Model file for the job. Use its own axes, mm. A direction names the side the tool comes from. Coordinates: 2 decimals unless noted, no trailing zeros. Write each loop counter-clockwise with the first axis right and the second up, starting at its lowest first coordinate (ties: lowest second). Pieces come first, ordered by that corner, then holes.
Q1. Pull direction Y, two halves, no side cores. Call faces 1 (the flat face through (1, 27, 228.6)), 2 (the cylindrical face through (24.6, 15.5, 11.2)), 3 (the flat face through (13, 50.8, 113)), 4 (the cylindrical face through (24.595, 35.423, 214.193)): released by +Y, released by -Y, zero draft, split by the parting line, or undercut.
Q2. Pin check, flat tip, straight feed: P1, Ø4, axis at y = 38.1, z = 215.9, coming from the -X side. Stop position of the tip, or through.
Q3. Drill centre lines: probe 1 along Z at (x, y) = (0.6, 38.1) (3 decimals); probe 2 along Y at (x, z) = (0.6, 12.7) (3 decimals); probe 3 along X at (y, z) = (37, 45). Where is each one in solid material? Low to high.
Q4. Band-saw the part on D-D, the plane x = 13.5. Write the cut outline in (y, z).
Q5. Band-saw the part on A-A, the plane y = 38.1. Write the cut outline in (x, z) (1 decimal), plus the area to 3 significant figures.
Q6. Band-saw the part on B-B, the plane z = 114.5. Write the cut outline in (x, y), plus the area to 3 significant figures.
Q7. Band-saw the part on C-C, the plane y = 25. Write the cut outline in (x, z), plus the area to 3 significant figures.
Q8. Which spindle directions (+Z, -Z, +X, -X, +Y, -Y) get a long thin tool onto all of the face, cutting with end or side? Do faces 5 (the flat face through (13, 0, 113)), 6 (the flat face through (1.588, 26, 113)). Say none if no direction does.
Autodesk Inventor part; units mm, degrees
ref_plane "YZ Plane" through (0, 0, 0) normal (1, 0, 0) x (0, 1, 0)
ref_plane "XZ Plane" through (0, 0, 0) normal (0, 1, 0) x (-1, 0, 0)
ref_plane "XY Plane" through (0, 0, 0) normal (0, 0, 1) x (1, 0, 0)
sketch "Sketch1" plane through (0, 0, 0) normal (0, 0, 1) x (1, 0, 0)
  line L0 (0, 0) -> (25.4, 0)
  line L1 (25.4, 0) -> (25.4, 50.8)
  line L2 (25.4, 50.8) -> (0, 50.8)
  line L3 (0, 50.8) -> (0, 0)
  dimension "d0" = 25.4
  dimension "d1" = 50.8
extrude "Extrusion1" add sketch "Sketch1" along normal blind 228.6
shell "Shell1" thickness 1.5875 removed faces 2 at (8.4667, 33.8667, 0) at (8.4667, 33.8667, 228.6)
hole "Hole1" at (25.4, 38.1, 215.9) direction (-1, 0, 0) diameter 6.35 end through all
hole "Hole2" at (25.4, 12.7, 215.9) direction (-1, 0, 0) diameter 6.35 end through all
hole "Hole3" at (25.4, 38.1, 12.7) direction (-1, 0, 0) diameter 6.35 end through all
hole "Hole4" at (25.4, 12.7, 12.7) direction (-1, 0, 0) diameter 6.35 end through all
properties part number "Flywheel Roller Right Side Support Beam"
Answer sheet:
1. face 1: zero draft
1. face 2: undercut
1. face 3: released by +Y
1. face 4: undercut
2. P1: passes through
3. probe 1: z = 0 to 9.525, 15.875 to 212.725, 219.075 to 228.6
3. probe 2: y = 0 to 9.525, 15.875 to 34.925, 41.275 to 50.8
3. probe 3: x = 0 to 1.59, 23.81 to 25.4
4. outline: (0, 0) - (1.59, 0) - (1.59, 228.6) - (0, 228.6) - close; (49.21, 0) - (50.8, 0) - (50.8, 228.6) - (49.21, 228.6) - close
5. outline: (0, 0) - (1.6, 0) - (1.6, 9.5) - (0, 9.5) - close; (0, 15.9) - (1.6, 15.9) - (1.6, 212.7) - (0, 212.7) - close; (0, 219.1) - (1.6, 219.1) - (1.6, 228.6) - (0, 228.6) - close; (23.8, 0) - (25.4, 0) - (25.4, 9.5) - (23.8, 9.5) - close; (23.8, 15.9) - (25.4, 15.9) - (25.4, 212.7) - (23.8, 212.7) - close; (23.8, 219.1) - (25.4, 219.1) - (25.4, 228.6) - (23.8, 228.6) - close
5. area: 685 mm2
6. outline: (0, 0) - (25.4, 0) - (25.4, 50.8) - (0, 50.8) - close; hole (1.59, 1.59) - (23.81, 1.59) - (23.81, 49.21) - (1.59, 49.21) - close
6. area: 232 mm2
7. outline: (0, 0) - (1.59, 0) - (1.59, 228.6) - (0, 228.6) - close; (23.81, 0) - (25.4, 0) - (25.4, 228.6) - (23.81, 228.6) - close
7. area: 726 mm2
8. face 5: +Z, -Z, +X, -X, -Y
8. face 6: +Z, -Z
